```python
from build123d import *

# Parameters (mm, degrees)
F0_W      = 25.4
F0_H      = 25.4
F1_DEPTH  = 7.62
F2_R      = 8.763
F3_DEPTH  = 19.431
F4_W      = 25.4
F4_H      = 25.4
F5_DEPTH  = 21.209
F6_R      = 6.35
F7_DEPTH  = 46.5582
F8_R      = 2.0828
F9_DEPTH  = 25.401
F11_DEPTH = 25.401
F13_DEPTH = 25.4
F14_R     = 2.0828
F15_DEPTH = 6.35


with BuildPart() as f1:
    # F0 (on Top) → F1 (new body)
    with BuildSketch(Plane.XY):
        Rectangle(F0_W, F0_H)
    extrude(amount=F1_DEPTH)

    # F2 (on face) → F3 (join)
    with BuildSketch(Plane.XY.offset(7.62)):
        Circle(F2_R)
    extrude(amount=F3_DEPTH)

    # F4 (on face) → F5 (join)
    with BuildSketch(Plane.XY.offset(27.051)):
        Rectangle(F4_W, F4_H)
    extrude(amount=F5_DEPTH)

    # F6 (on face) → F7 (cut)
    with BuildSketch(Plane(origin=(0, 0, 0), x_dir=(1, 0, 0), z_dir=(0, 0, -1))):
        Circle(F6_R)
    extrude(amount=-F7_DEPTH, mode=Mode.SUBTRACT)

    # F8 (on face) → F9 (cut, through all)
    with BuildSketch(Plane.XZ.offset(12.7)):
        with Locations((-9.525, 45.085)):
            Circle(F8_R)
        with Locations((9.525, 45.085)):
            Circle(F8_R)
        with Locations((-9.525, 30.226)):
            Circle(F8_R)
        with Locations((9.525, 30.226)):
            Circle(F8_R)
    extrude(amount=-F9_DEPTH, mode=Mode.SUBTRACT)

    # F10 (on face) → F11 (cut, through all)
    with BuildSketch(Plane(origin=(0, 12.7, 0), x_dir=(-1, 0, 0), z_dir=(0, 1, 0))):
        with BuildLine():
            ThreePointArc((7.9375, 37.6555), (5.6126600757, 43.2681600757), (0, 45.593))
            Line((0, 45.593), (0, 29.718))
            ThreePointArc((0, 29.718), (5.6126600757, 32.0428399243), (7.9375, 37.6555))
        make_face()
        with BuildLine():
            Line((0, 29.718), (0, 45.593))
            ThreePointArc((0, 45.593), (-7.9375, 37.6555), (0, 29.718))
        make_face()
    extrude(amount=-F11_DEPTH, mode=Mode.SUBTRACT)

    # F12 (on Front) → F13 (cut)
    with BuildSketch(Plane.XZ):
        with BuildLine():
            Line((-1.5875, 12.3317), (0, 12.3317))
            Line((0, 12.3317), (0, 13.9192))
            ThreePointArc((0, 13.9192), (-0.4649679849, 12.7966679849), (-1.5875, 12.3317))
        make_face()
        with BuildLine():
            Line((0, 13.9192), (0, 12.3317))
            Line((0, 12.3317), (1.5875, 12.3317))
            ThreePointArc((1.5875, 12.3317), (0.4649679849, 12.7966679849), (0, 13.9192))
        make_face()
        with BuildLine():
            ThreePointArc((1.5875, 15.5067), (0.4649679849, 15.0417320151), (0, 13.9192))
            Line((0, 13.9192), (1.5875, 13.9192))
            Line((1.5875, 13.9192), (1.5875, 15.5067))
        make_face()
        with BuildLine():
            ThreePointArc((-1.5875, 15.5067), (-0.4649679849, 15.0417320151), (0, 13.9192))
            ThreePointArc((0, 13.9192), (0.4649679849, 15.0417320151), (1.5875, 15.5067))
            Line((1.5875, 15.5067), (-1.5875, 15.5067))
        make_face()
        with BuildLine():
            Line((1.5875, 13.9192), (0, 13.9192))
            ThreePointArc((0, 13.9192), (0.4649679849, 12.7966679849), (1.5875, 12.3317))
            Line((1.5875, 12.3317), (1.5875, 13.9192))
        make_face()
        with BuildLine():
            ThreePointArc((-1.5875, 12.3317), (-0.4649679849, 12.7966679849), (0, 13.9192))
            ThreePointArc((0, 13.9192), (-0.4649679849, 15.0417320151), (-1.5875, 15.5067))
            ThreePointArc((-1.5875, 15.5067), (-3.175, 13.9192), (-1.5875, 12.3317))
        make_face()
        with BuildLine():
            Line((1.5875, 13.9192), (1.5875, 12.3317))
            ThreePointArc((1.5875, 12.3317), (2.7100320151, 12.7966679849), (3.175, 13.9192))
            ThreePointArc((3.175, 13.9192), (2.7100320151, 15.0417320151), (1.5875, 15.5067))
            Line((1.5875, 15.5067), (1.5875, 13.9192))
        make_face()
    extrude(amount=-F13_DEPTH, mode=Mode.SUBTRACT)

    # F14 (on face) → F15 (cut)
    with BuildSketch(Plane(origin=(0, 0, 0), x_dir=(1, 0, 0), z_dir=(0, 0, -1))):
        with Locations((-9.525, 9.525)):
            Circle(F14_R)
        with Locations((-9.525, -9.525)):
            Circle(F14_R)
        with Locations((9.525, 9.525)):
            Circle(F14_R)
        with Locations((9.525, -9.525)):
            Circle(F14_R)
    extrude(amount=-F15_DEPTH, mode=Mode.SUBTRACT)


solid = f1.part
```
The listing builds one solid part. Answer for the finished solid, in the listing's coordinates (mm). A direction names the side the tool comes from. Round coordinates to 2 decimals unless told otherwise and drop trailing zeros. Loops run counter-clockwise (first coordinate to the right, second up) from the corner with the lowest first, then second, coordinate; pieces in that order, holes last. Notation, with made-up numbers: (9.5, 58) - (13.5, 58) arc R28 cw to (13.5, 96) - close; hole circle Ø4 at (70, 19.25). An arc over 180 degrees is marked (long way). Use one line per item in the form item = value. Start each with the question number.
1. Consider line 1 (Z direction, x = 9.75, y = -8); line 2 (X direction, y = -4, z = 43.5); line 3 (Z direction, x = -8.5, y = 10.5). Determine where each line is inside the solid, lowest interval first. Write a range as [from, to].
2. The part is cut by section C-C on z = 17. Determine the outline of the cut face in (x, y), then the cut area to 3 significant figures.
3. The part is cut by section D-D on x = -1. Determine the outline of the cut face in (y, z), then the cut area to 3 significant figures.
4. A tool of negligible diameter and unlimited length cuts with its end or side. For faces 1 (the face through (0, 12.7, 4)), 2 (the face through (0, 7, 12.332)), 3 (the face through (-3, 9, 7.62)), 4 (the face through (6.057, -1.907, 44.919)), 5 (the face through (10.49, -0.18, 28.38)), from which of +Z, -Z, +X, -X, +Y, -Y can it reach the whole face along a straight path? Write none if from no direction.
5. The part is cut by section A-A on y = 1. Determine the outline of the cut face in (x, z) (1 decimal), then the cut area to 3 significant figures.
6. The part is cut by section B-B on x = -5. Determine the outline of the cut face in (y, z), then the cut area to 3 significant figures.
7. Given pin 1 Ø1.5 at (x, z) = (-6, 39.5) entering from -Y; pin 2 Ø10 at (y, z) = (-2.5, 20.5) entering from -X; pin 3 Ø2 at (x, y) = (9.5, -10.5) entering from -Z; pin 4 Ø6 at (y, z) = (7, 11) entering from -X, each flat-ended and moving along its own axis, determine where each tip first touches the part or whether it passes through.
8. For a pull along X with two mould halves and no side action, classify faces 6 (the face through (-10, 9, 6.35)), 7 (the face through (-3, 6, 0)), 8 (the face through (12.7, 0, 38)), 9 (the face through (-1.9, -8.555, 17.199)) as pulls with the +X half, pulls with the -X half, needs draft (parallel to the pull), parting line crosses it, or undercut.
Geometry check:
q1.line_1 = [6.35, 7.62], [27.05, 28.16], [32.3, 43.01], [47.16, 48.26]
q1.line_2 = [-12.7, -10.88], [-8.17, -5.37], [5.37, 8.17], [10.88, 12.7]
q1.line_3 = [6.35, 7.62], [27.05, 28.41], [32.04, 43.27], [46.9, 48.26]
q2.outline = circle Ø17.53 at (0, 0); hole circle Ø12.7 at (0, 0)
q2.area = 115 mm^2
q3.outline = (-12.7, 0) - (-6.27, 0) - (-6.27, 29.78) - (-12.7, 29.78) - (-12.7, 27.05) - (-8.71, 27.05) - (-8.71, 7.62) - (-12.7, 7.62) - close; (-12.7, 45.53) - (-6.27, 45.53) - (-6.27, 46.56) - (6.27, 46.56) - (6.27, 45.53) - (12.7, 45.53) - (12.7, 48.26) - (-12.7, 48.26) - close; (6.27, 0) - (12.7, 0) - (12.7, 7.62) - (8.71, 7.62) - (8.71, 12.33) - (6.27, 12.33) - close; (6.27, 15.51) - (8.71, 15.51) - (8.71, 27.05) - (12.7, 27.05) - (12.7, 29.78) - (6.27, 29.78) - close
q3.area = 276 mm^2
q4.face_1 = +Z, -Z, +X, -X, +Y
q4.face_2 = +Y
q4.face_3 = none
q4.face_4 = -Z
q4.face_5 = +Y, -Y
q5.outline = (-12.7, 0) - (-6.3, 0) - (-6.3, 32.8) arc R7.9 cw to (-6.3, 42.5) - (-6.3, 46.6) - (6.3, 46.6) - (6.3, 42.5) arc R7.9 cw to (6.3, 32.8) - (6.3, 0) - (12.7, 0) - (12.7, 7.6) - (8.7, 7.6) - (8.7, 27.1) - (12.7, 27.1) - (12.7, 48.3) - (-12.7, 48.3) - (-12.7, 27.1) - (-8.7, 27.1) - (-8.7, 7.6) - (-12.7, 7.6) - close; hole circle Ø4.2 at (-9.5, 30.2); hole circle Ø4.2 at (-9.5, 45.1); hole circle Ø4.2 at (9.5, 30.2); hole circle Ø4.2 at (9.5, 45.1)
q5.area = 410 mm^2
q6.outline = (-12.7, 0) - (-3.91, 0) - (-3.91, 31.49) - (-12.7, 31.49) - (-12.7, 27.05) - (-7.2, 27.05) - (-7.2, 7.62) - (-12.7, 7.62) - close; (-12.7, 43.82) - (-3.91, 43.82) - (-3.91, 46.56) - (3.91, 46.56) - (3.91, 43.82) - (12.7, 43.82) - (12.7, 48.26) - (-12.7, 48.26) - close; (3.91, 0) - (12.7, 0) - (12.7, 7.62) - (7.2, 7.62) - (7.2, 27.05) - (12.7, 27.05) - (12.7, 31.49) - (3.91, 31.49) - close
q6.area = 431 mm^2
q7.pin_1 = through
q7.pin_2 = -8.76
q7.pin_3 = 6.35
q7.pin_4 = -7.8
q8.face_6 = undercut
q8.face_7 = needs draft
q8.face_8 = pulls with the +X half
q8.face_9 = parting line crosses it
